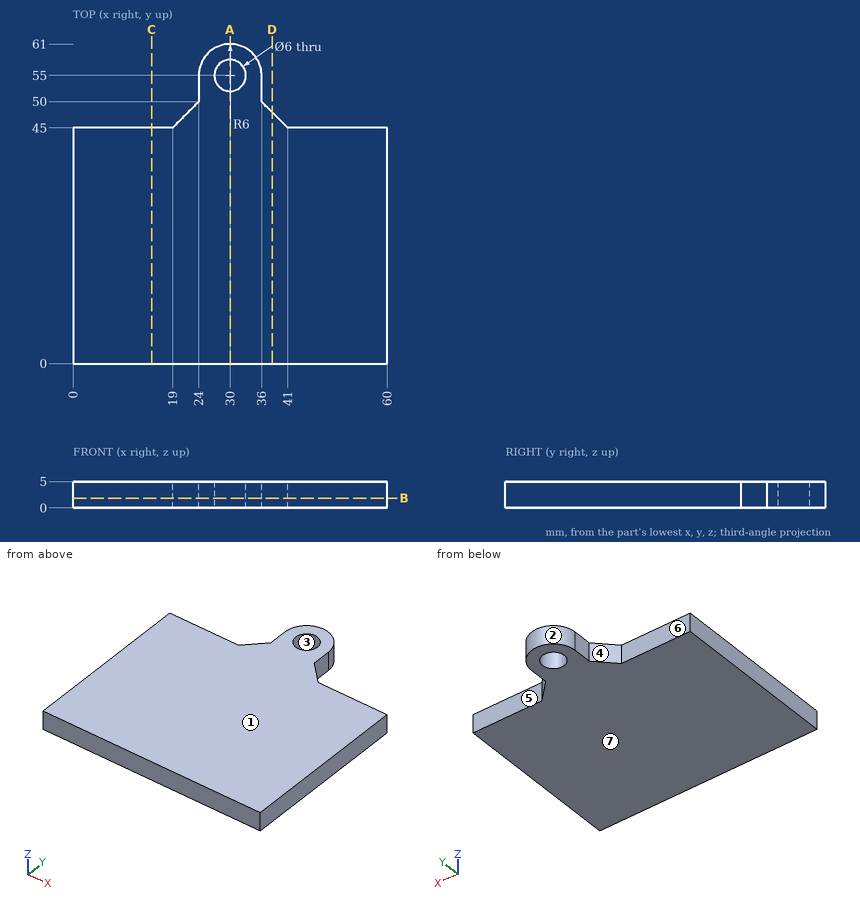
Input: dimensioned drawing with shaded views. Units: mm. Origin: part minimum x, y, z. A direction names the side the tool comes from. Give positions to 0.01 mm unless a question says otherwise; leave off trailing zeros. Write each loop counter-clockwise with the first axis right and the second up, starting at its lowest first coordinate (ties: lowest second). Pieces come first, ordered by that corner, then holes. Notation, with made-up numbers: (-31, -12) - (14, -12) arc R11 ccw to (14, 0) - close; hole circle Ø7 at (-21.75, 43). An arc over 180 degrees is marked (long way). Write item = value, one per line. Start each with the question number.
1) Cut plane C-C (x = 15). Return loops of the section in (y, z), and give its area (3 significant figures).
2) Pin query (flat end, axial travel): pin 1 (2.5 mm diameter, centred on y = 51.5, z = 2.5, fed in from -X); pin 2 (2.5 mm diameter, centred on y = 53.5, z = 2, fed in from +X); pin 3 (2.5 mm diameter, centred on x = 10, z = 2, fed in from +Y); pin 4 (5.5 mm diameter, centred on x = 30, y = 55, fed in from -Z). Return the tip coordinate at first contact, or that it passes through.
3) Material intervals for L1, parallel to Y at x = 30, z = 2.4; L2, parallel to Y at x = 54.5, z = 2.7, sorted ascending. Write a range as [from, to].
4) Cut plane A-A (x = 30). Return loops of the section in (y, z).
5) Cut plane D-D (x = 38). Return loops of the section in (y, z).
6) Cut plane B-B (z = 1.85). Return loops of the section in (x, y), and give its area (3 significant figures).
7) Reachability of the marked faces 5, 6 and 7 from +Z, -Z, +X, -X, +Y, -Y: full face, straight path, thin tool, end or side. Return the list, or none.
8) Draft query along X for the marked faces 1, 2, 3 and 4. Return one class per face: pulls with the +X half, pulls with the -X half, needs draft (parallel to the pull), parting line crosses it, or undercut.
Answers follow:
q1.outline = (0, 0) - (45, 0) - (45, 5) - (0, 5) - close
q1.area = 225 mm^2
q2.pin_1 = 24
q2.pin_2 = 36
q2.pin_3 = 45
q2.pin_4 = through
q3.L1 = [0, 52], [58, 61]
q3.L2 = [0, 45]
q4.outline = (0, 0) - (52, 0) - (52, 5) - (0, 5) - close; (58, 0) - (61, 0) - (61, 5) - (58, 5) - close
q5.outline = (0, 0) - (48, 0) - (48, 5) - (0, 5) - close
q6.outline = (0, 0) - (60, 0) - (60, 45) - (41, 45) - (36, 50) - (36, 55) arc R6 ccw to (24, 55) - (24, 50) - (19, 45) - (0, 45) - close; hole circle Ø6 at (30, 55)
q6.area = 2,870 mm^2
q7.face_5 = +Z, -Z, +X, +Y
q7.face_6 = +Z, -Z, -X, +Y
q7.face_7 = -Z, +X, -X, +Y, -Y
q8.face_1 = needs draft
q8.face_2 = parting line crosses it
q8.face_3 = undercut
q8.face_4 = pulls with the -X half
